from build123d import *

# Parameters (mm, degrees)
BOSS_EXTRUDE1_DEPTH            = 30
SKETCH2_R                      = 2.6
SKETCH2_R_2                    = 1.55
BOSS_EXTRUDE3_DEPTH            = 5
CUT_EXTRUDE1_REACH             = 90.931
CUT_EXTRUDE1_DIRECTION_2_DEPTH = 89.931178746
CUT_EXTRUDE2_REACH             = 90.931
CUT_EXTRUDE2_DIRECTION_2_DEPTH = 89.931178746
FILLET1_R                      = 2
SKETCH6_R                      = 2.6
BOSS_EXTRUDE4_DEPTH            = 1


with BuildPart() as part:
    # Sketch1 → Boss-Extrude1 (new body)
    with BuildSketch(Plane(origin=(0, 0, 0), x_dir=(1, 0, 0), z_dir=(0, 1, 0))):
        Polygon((-13.5, 0), (0, 74.39897269), (13.5, 0), (14.483932895, 0.178538676), (0, 80), (-14.483932895, 0.178538676), align=None)
    extrude(amount=BOSS_EXTRUDE1_DEPTH)

    # Sketch2 → Boss-Extrude3 (add)
    # profile 1 of 8: a face of its own
    with BuildSketch(Plane(origin=(0, 0, 0), x_dir=(1, 0, 0), z_dir=(0, 1, 0))):
        with Locations((11.925707369, -0.285661882)):
            Circle(SKETCH2_R)
        with Locations(Location((11.925707369, -0.285661882, 0), (0, 0, 270))):
            Circle(SKETCH2_R_2, mode=Mode.SUBTRACT)
    # profile 2 of 8: a face of its own
    with BuildSketch(Plane(origin=(0, 0, 0), x_dir=(1, 0, 0), z_dir=(0, 1, 0))):
        with Locations((9.426165905, 13.489398644)):
            Circle(SKETCH2_R)
        with Locations(Location((9.426165905, 13.489398644, 0), (0, 0, 270))):
            Circle(SKETCH2_R_2, mode=Mode.SUBTRACT)
    # profile 3 of 8: a face of its own
    with BuildSketch(Plane(origin=(0, 0, 0), x_dir=(1, 0, 0), z_dir=(0, 1, 0))):
        with Locations((6.926624441, 27.264459169)):
            Circle(SKETCH2_R)
        with Locations(Location((6.926624441, 27.264459169, 0), (0, 0, 270))):
            Circle(SKETCH2_R_2, mode=Mode.SUBTRACT)
    # profile 4 of 8: a face of its own
    with BuildSketch(Plane(origin=(0, 0, 0), x_dir=(1, 0, 0), z_dir=(0, 1, 0))):
        with Locations((4.427082978, 41.039519694)):
            Circle(SKETCH2_R)
        with Locations(Location((4.427082978, 41.039519694, 0), (0, 0, 270))):
            Circle(SKETCH2_R_2, mode=Mode.SUBTRACT)
    # profile 5 of 8: a face of its own
    with BuildSketch(Plane(origin=(0, 0, 0), x_dir=(1, 0, 0), z_dir=(0, 1, 0))):
        with Locations((-11.925707369, -0.285661882)):
            Circle(SKETCH2_R)
        with Locations(Location((-11.925707369, -0.285661882, 0), (0, 0, 90))):
            Circle(SKETCH2_R_2, mode=Mode.SUBTRACT)
    # profile 6 of 8: a face of its own
    with BuildSketch(Plane(origin=(0, 0, 0), x_dir=(1, 0, 0), z_dir=(0, 1, 0))):
        with Locations((-9.426165905, 13.489398644)):
            Circle(SKETCH2_R)
        with Locations(Location((-9.426165905, 13.489398644, 0), (0, 0, 90))):
            Circle(SKETCH2_R_2, mode=Mode.SUBTRACT)
    # profile 7 of 8: a face of its own
    with BuildSketch(Plane(origin=(0, 0, 0), x_dir=(1, 0, 0), z_dir=(0, 1, 0))):
        with Locations((-6.926624441, 27.264459169)):
            Circle(SKETCH2_R)
        with Locations(Location((-6.926624441, 27.264459169, 0), (0, 0, 90))):
            Circle(SKETCH2_R_2, mode=Mode.SUBTRACT)
    # profile 8 of 8: a face of its own
    with BuildSketch(Plane(origin=(0, 0, 0), x_dir=(1, 0, 0), z_dir=(0, 1, 0))):
        with Locations((-4.427082978, 41.039519694)):
            Circle(SKETCH2_R)
        with Locations(Location((-4.427082978, 41.039519694, 0), (0, 0, 90))):
            Circle(SKETCH2_R_2, mode=Mode.SUBTRACT)
    boss_extrude3 = extrude(amount=BOSS_EXTRUDE3_DEPTH)

    # Cut-Extrude1: up to this face of the body (flat: up to its plane)
    cut_extrude1_end = Plane(part.part.faces().sort_by_distance((-6.670361164, 15.408163761, -37.638378758))[0])
    # Sketch4 → Cut-Extrude1 (cut, up to the picked face)
    with BuildSketch(Plane(origin=(0.430326794, 0, 2.371546029), x_dir=(0.9839328946538309, 0, -0.17853867597283662), z_dir=(0.17853867597283662, 0, 0.9839328946538309)), mode=Mode.PRIVATE) as cut_extrude1_sk1:
        Polygon((13.283094078, 5), (9.083094078, 5), (9.083094078, 1.475781549), align=None)
    cut_extrude1_tool1 = split(extrude(cut_extrude1_sk1.sketch, amount=-CUT_EXTRUDE1_REACH, mode=Mode.PRIVATE), bisect_by=cut_extrude1_end, keep=Keep.BOTH, mode=Mode.PRIVATE)
    cut_extrude1 = cut_extrude1_tool1.solids().sort_by(Axis((10.744988, 3.825261, 0.499908), (-0.17853867597283662, 0, -0.9839328946538309)))[0]
    add(cut_extrude1, mode=Mode.SUBTRACT)

    # Sketch4 → Cut-Extrude1 direction 2 (cut)
    with BuildSketch(Plane(origin=(0.430326794, 0, 2.371546029), x_dir=(0.9839328946538309, 0, -0.17853867597283662), z_dir=(0.17853867597283662, 0, 0.9839328946538309))):
        Polygon((13.283094078, 5), (9.083094078, 5), (9.083094078, 1.475781549), align=None)
    cut_extrude1_direction_2 = extrude(amount=CUT_EXTRUDE1_DIRECTION_2_DEPTH, mode=Mode.SUBTRACT)

    # Cut-Extrude2: up to this face of the body (flat: up to its plane)
    cut_extrude2_end = Plane(part.part.faces().sort_by_distance((6.670361164, 15.408163761, -37.638378758))[0])
    # Sketch5 → Cut-Extrude2 (cut, up to the picked face)
    with BuildSketch(Plane(origin=(-0.430326794, 0, 2.371546029), x_dir=(0.9839328946538308, 0, 0.17853867597283732), z_dir=(-0.17853867597283732, 0, 0.9839328946538308)), mode=Mode.PRIVATE) as cut_extrude2_sk1:
        Polygon((-9.083094078, 5), (-9.083094078, 1.475781549), (-13.283094078, 5), align=None)
    cut_extrude2_tool1 = split(extrude(cut_extrude2_sk1.sketch, amount=-CUT_EXTRUDE2_REACH, mode=Mode.PRIVATE), bisect_by=cut_extrude2_end, keep=Keep.BOTH, mode=Mode.PRIVATE)
    cut_extrude2 = cut_extrude2_tool1.solids().sort_by(Axis((-10.744988, 3.825261, 0.499908), (0.17853867597283732, 0, -0.9839328946538308)))[0]
    add(cut_extrude2, mode=Mode.SUBTRACT)

    # Sketch5 → Cut-Extrude2 direction 2 (cut)
    with BuildSketch(Plane(origin=(-0.430326794, 0, 2.371546029), x_dir=(0.9839328946538308, 0, 0.17853867597283732), z_dir=(-0.17853867597283732, 0, 0.9839328946538308))):
        Polygon((-9.083094078, 5), (-9.083094078, 1.475781549), (-13.283094078, 5), align=None)
    cut_extrude2_direction_2 = extrude(amount=CUT_EXTRUDE2_DIRECTION_2_DEPTH, mode=Mode.SUBTRACT)

    # Mirror2: Boss-Extrude3, Cut-Extrude1, Cut-Extrude1 direction 2, Cut-Extrude2, Cut-Extrude2 direction 2 across plane
    add(boss_extrude3.mirror(Plane.ZX.offset(15)))
    add(cut_extrude1.mirror(Plane.ZX.offset(15)), mode=Mode.SUBTRACT)
    add(cut_extrude1_direction_2.mirror(Plane.ZX.offset(15)), mode=Mode.SUBTRACT)
    add(cut_extrude2.mirror(Plane.ZX.offset(15)), mode=Mode.SUBTRACT)
    add(cut_extrude2_direction_2.mirror(Plane.ZX.offset(15)), mode=Mode.SUBTRACT)

    # Fillet1
    # the kernel refuses this fillet: 2 mm, written as the material it adds along each edge
    with BuildSketch(Plane(origin=(13.5, 5, 0), x_dir=(0, 1, 0), z_dir=(0.9839328946538308, 0, -0.17853867597283668))) as fillet1_piece_1_section:
        with BuildLine():
            CenterArc((FILLET1_R, FILLET1_R), FILLET1_R, 180, 90)
            Line((0, FILLET1_R), (0, 0))
            Line((0, 0), (FILLET1_R, 0))
        make_face()
    fillet1_piece_1 = extrude(amount=6, mode=Mode.PRIVATE)
    fillet1_piece_1 = fillet1_piece_1 & Plane(origin=(11.925707369, 5.699977742, 0.285661882), x_dir=(1, 0, 0), z_dir=(0, -1, 0)) * Cylinder(2.6, 20, mode=Mode.PRIVATE)
    add(fillet1_piece_1)
    with BuildSketch(Plane(origin=(13.5, 25, 0), x_dir=(0, -1, 0), z_dir=(0.9839328946538308, 0, -0.17853867597283668))) as fillet1_piece_2_section:
        with BuildLine():
            CenterArc((FILLET1_R, -FILLET1_R), FILLET1_R, 90, 90)
            Line((0, -FILLET1_R), (0, 0))
            Line((0, 0), (FILLET1_R, 0))
        make_face()
    fillet1_piece_2 = extrude(amount=6, mode=Mode.PRIVATE)
    fillet1_piece_2 = fillet1_piece_2 & Plane(origin=(11.925707369, 24.300022258, 0.285661882), x_dir=(1, 0, 0), z_dir=(0, 1, 0)) * Cylinder(2.6, 20, mode=Mode.PRIVATE)
    add(fillet1_piece_2)
    with BuildSketch(Plane(origin=(-19.403597368, 25, -1.071232056), x_dir=(0, -1, 0), z_dir=(0.9839328946538307, 0, 0.17853867597283735))) as fillet1_piece_3_section:
        with BuildLine():
            CenterArc((FILLET1_R, -FILLET1_R), FILLET1_R, 90, 90)
            Line((0, -FILLET1_R), (0, 0))
            Line((0, 0), (FILLET1_R, 0))
        make_face()
    fillet1_piece_3 = extrude(amount=6, mode=Mode.PRIVATE)
    fillet1_piece_3 = fillet1_piece_3 & Plane(origin=(-11.925707369, 24.777637105, 0.285661882), x_dir=(1, 0, 0), z_dir=(0, 1, 0)) * Cylinder(2.6, 21, mode=Mode.PRIVATE)
    add(fillet1_piece_3)
    with BuildSketch(Plane(origin=(-19.403597368, 5, -1.071232056), x_dir=(-0.17853867597283735, 0, 0.9839328946538307), z_dir=(0.9839328946538307, 0, 0.17853867597283735))) as fillet1_piece_4_section:
        with BuildLine():
            CenterArc((FILLET1_R, -FILLET1_R), FILLET1_R, 90, 90)
            Line((0, -FILLET1_R), (0, 0))
            Line((0, 0), (FILLET1_R, 0))
        make_face()
    fillet1_piece_4 = extrude(amount=6, mode=Mode.PRIVATE)
    fillet1_piece_4 = fillet1_piece_4 & Plane(origin=(-11.925707369, 5.222362792, 0.285661882), x_dir=(1, 0, 0), z_dir=(0, -1, 0)) * Cylinder(2.6, 21, mode=Mode.PRIVATE)
    add(fillet1_piece_4)

    # Sketch6 → Boss-Extrude4 (add)
    with BuildSketch(Plane.XZ):
        with Locations((4.427082978, -41.039519694)):
            Circle(SKETCH6_R)
        with Locations((-4.427082978, -41.039519694)):
            Circle(SKETCH6_R)
        with Locations((-6.926624441, -27.264459169)):
            Circle(SKETCH6_R)
        with Locations((11.925707369, 0.285661882)):
            Circle(SKETCH6_R)
        with Locations((6.926624441, -27.264459169)):
            Circle(SKETCH6_R)
        with Locations((9.426165905, -13.489398644)):
            Circle(SKETCH6_R)
        with Locations((-9.426165905, -13.489398644)):
            Circle(SKETCH6_R)
        with Locations((-11.925707369, 0.285661882)):
            Circle(SKETCH6_R)
    extrude(amount=-BOSS_EXTRUDE4_DEPTH)


solid = part.part
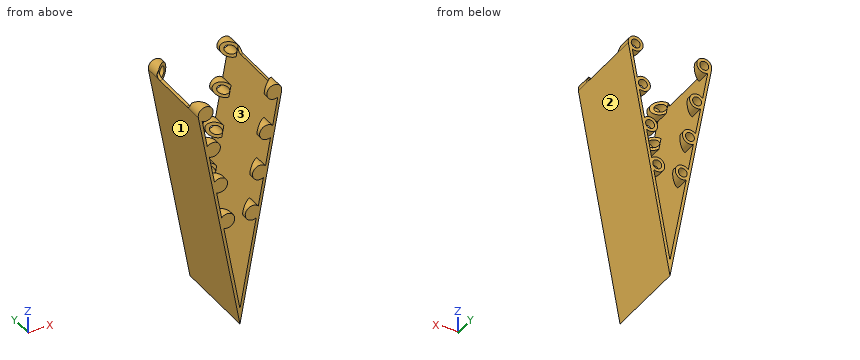
The listing builds one solid part. Answer for the finished solid, in the listing's coordinates (mm). Face numbers are marked on the shaded views. Round coordinates to 2 decimals unless told otherwise and drop trailing zeros. Write each loop counter-clockwise with the first axis right and the second up, starting at its lowest first coordinate (ties: lowest second). Pieces come first, ordered by that corner, then holes. Notation, with made-up numbers: M -15.75,78.25 L 13.25,78.25 A31 cw 13.25,103.25 Z; hole C 15,-1 d7. An arc over 180 degrees is marked long. Write each question's results on one line, items separated by ' | '. Start each with the question number.
Item 1: Find section C-C on y = 6. Write down the section's boundary in (x, z), and give its area (3 significant figures).
Item 2: Find section B-B on y = 9.5. Write down the section's boundary in (x, z).
Item 3: Find section A-A on z = -52. Write down the section's boundary in (x, y), and give its area (3 significant figures).
Item 4: Given pin 1 Ø5 at (x, z) = (-7, -66.5) entering from -Y; pin 2 Ø1.6 at (x, z) = (12, 0) entering from +Y; pin 3 Ø3 at (y, z) = (21, -11) entering from -X; pin 4 Ø2 at (y, z) = (17.5, -28.5) entering from -X, each flat-ended and moving along its own axis, determine where each tip first touches the part or whether it passes through.
Item 5: The mould has two halves that part along X. Classify the marked faces 1, 2 and 3: +X half, -X half, draft (parallel to the pull), parting line (faces both ways), or undercut.
Item 6: Straight lines are drawn through the part: probe 1 along X at (y, z) = (10.5, -38.5); probe 2 along X at (y, z) = (19, -21); probe 3 along Y at (x, z) = (-2, -40.5). For each, find the intervals that lie inside material, in ascending order.
Answer block:
1) outline: M -14.52,0.09 A2.6 ccw -14.48,-0.18 L 0,-80 L 14.48,-0.18 A2.6 ccw 14.52,0.09 L 13.55,0.26 L 0,-74.4 L -13.55,0.26 Z | area: 157 mm²
2) outline: M -14.48,-0.18 L 0,-80 L 14.48,-0.18 L 13.5,0 L 0,-74.4 L -13.5,0 Z
3) outline: M -5.08,0 L -4.06,0 L -4.06,30 L -5.08,30 Z; M 4.06,0 L 5.08,0 L 5.08,30 L 4.06,30 Z | area: 61.0 mm²
4) pin 1: passes through | pin 2: stops at y = 1 | pin 3: stops at x = -12.79 | pin 4: stops at x = -9.53
5) face 1: -X half | face 2: +X half | face 3: undercut
6) probe 1: x = -7.53 to -6.51, 6.51 to 7.53 | probe 2: x = -10.71 to -9.69, 9.69 to 10.71 | probe 3: y = 0 to 1.57, 28.43 to 30
